CAD build for the part. Positions are in the model's coordinates, mm. A direction names the side the tool comes from. Give positions to 0.01 mm unless a question says otherwise; leave off trailing zeros. Loops run counter-clockwise (first coordinate to the right, second up) from the corner with the lowest first, then second, coordinate; pieces in that order, holes last. Notation, with made-up numbers: (34, -21) -> (40, -21) arc R20 cw to (40, 10) -> close; hole circle Ø10 at (-40, 18). An arc over 180 degrees is marked (long way). Use one line per item in the form item = value.
```python
from build123d import *

# Parameters (mm, degrees)
F0_R     = 3.75
F1_DEPTH = 25
F2_R     = 7.5
F3_DEPTH = 2
F4_R     = 0.6
F5_SIZE  = 0.6


with BuildPart() as f1:
    # F0 (on Front) → F1 (new body)
    with BuildSketch(Plane.XZ):
        Circle(F0_R)
    extrude(amount=F1_DEPTH)

    # F2 (on Front) → F3 (join)
    with BuildSketch(Plane.XZ):
        Circle(F2_R)
    extrude(amount=F3_DEPTH)

    # F4
    f4_edges = [f1.edges().sort_by_distance(p)[0] for p in [
        (-7.5, 0, 0),
    ]]
    fillet(f4_edges, radius=F4_R)

    # F5
    f5_edges = [f1.edges().sort_by_distance(p)[0] for p in [
        (-3.75, -25, 0),
    ]]
    chamfer(f5_edges, length=F5_SIZE)


solid = f1.part
```
1. Cut at C-C, the plane y = -4.5. Write the cut outline in (x, z).
Result sheet:
outline = circle Ø7.5 at (0, 0)
2. Tool access for faces 1 (the flat face through (0, 0, 0)), 2 (the flat face through (3, -2, -3)): list every direction of +Z, -Z, +X, -X, +Y, -Y with a clear straight run to the whole face (end or side of a thin tool).
Result sheet:
face_1 = +Z, -Z, +X, -X, +Y
face_2 = -Y
3. Drop flat-ended pins along their axis: P1, Ø5, axis at x = -4, z = 0.5, coming from the -Y side; P2, Ø1.5, axis at x = -4.5, z = -3, coming from the -Y side; P3, Ø6, axis at x = 2.5, y = -10.5, coming from the +Z side; P4, Ø1, axis at x = -4.5, y = -21.5, coming from the -Z side. Give the stop position or say it passes through.
Result sheet:
P1 = -25
P2 = -2
P3 = 3.75
P4 = through
4. Cut at A-A, the plane z = 0. Write the cut outline in (x, y), then the cut area to 3 significant figures.
Result sheet:
outline = (-7.5, -2) -> (-3.75, -2) -> (-3.75, -24.4) -> (-3.15, -25) -> (3.15, -25) -> (3.75, -24.4) -> (3.75, -2) -> (7.5, -2) -> (7.5, -0.6) arc R0.6 ccw to (6.9, 0) -> (-6.9, 0) arc R0.6 ccw to (-7.5, -0.6) -> close
area = 202 mm^2
5. Cut at B-B, the plane x = 0. Write the cut outline in (y, z), then the cut area to 3 significant figures.
Result sheet:
outline = (-25, -3.15) -> (-24.4, -3.75) -> (-2, -3.75) -> (-2, -7.5) -> (-0.6, -7.5) arc R0.6 ccw to (0, -6.9) -> (0, 6.9) arc R0.6 ccw to (-0.6, 7.5) -> (-2, 7.5) -> (-2, 3.75) -> (-24.4, 3.75) -> (-25, 3.15) -> close
area = 202 mm^2
6. Drill centre lines: line 1 (Y direction, x = 4.5, z = 5.25); line 2 (Z direction, x = 5, y = -1.25); line 3 (X direction, y = -7.25, z = -3.25). Where is each one in solid material? Low to high.
Result sheet:
line_1 = -2 to 0
line_2 = -5.59 to 5.59
line_3 = -1.87 to 1.87
